```python
from build123d import *

# Parameters (mm, degrees)
F0_W     = 400
F0_H     = 1000
F0_W_2   = 250
F0_H_2   = 625
F0_H_3   = 150
F1_DEPTH = 50
F3_DEPTH = 400


with BuildPart() as f1:
    # F0 (on Front) → F1 (new body)
    with BuildSketch(Plane.XZ):
        with Locations((200, -500)):
            Rectangle(F0_W, F0_H)
        with Locations((200, -587.5)):
            Rectangle(F0_W_2, F0_H_2, mode=Mode.SUBTRACT)
        with Locations((200, -150)):
            Rectangle(F0_W_2, F0_H_3, mode=Mode.SUBTRACT)
    extrude(amount=-F1_DEPTH)

    # F2 (on face) → F3 (join)
    with BuildSketch(Plane.YZ.offset(400)):
        Polygon((-70, -1000), (0, -1000), (0, -962.657111), (-70, -975), align=None)
    extrude(amount=-F3_DEPTH)


solid = f1.part
```
Design review of the part built by this model. Coordinates are the model's own, in mm. A direction names the side the tool comes from. Give positions to 0.01 mm unless a question says otherwise; leave off trailing zeros. Order: outer loops, then holes, each group sorted by start corner. A loop starts at its lowest first (then second) coordinate and runs counter-clockwise, first axis right, second up. Notation, with made-up numbers: M 27.25,-20 L 75.25,-20 A37 ccw 75.25,16 Z; hole C 36,42.5 d2. An arc over 180 degrees is marked long. One line per question, with ' | ' between items. Start each with the question number.
Q1. The part is to be moulded in two halves that separate along X. For faces 4 (the face through (197, 25, 0)), 5 (the face through (0, 16, -493)), 6 (the face through (198, 25, -900)), say which applies: +X half, -X half, draft (parallel to the pull), parting line (faces both ways), or undercut.
Q2. For pin 1 Ø3 at (x, y) = (82.5, -58) entering from +Z; pin 2 Ø6 at (x, z) = (341, -542.5) entering from -Y; pin 3 Ø5 at (x, y) = (240, -28.5) entering from +Z, all flat-tipped, find the tip position at first contact; note any pin that passes through.
Q3. We need section A-A (z = -462.5). Write out the cut boundary in (x, y), plus the area to 3 significant figures.
Q4. Machinability: for faces 1 (the face through (400, 16, -493)), 2 (the face through (198, 25, -225)), 3 (the face through (331, 0, -475)), which of the approach directions +Z, -Z, +X, -X, +Y, -Y give a long, thin tool a straight path to every point of the face, cutting with its end or side? Answer none if there is none.
Q5. We need section D-D (x = 55). Write out the cut boundary in (y, z).
Q6. We need section B-B (y = 11.5). Write out the cut boundary in (x, z).
Q7. We need section C-C (x = 177). Write out the cut boundary in (y, z), plus the area to 3 significant figures.
Q8. For L1, parallel to Z at x = 285, y = 23.5; L2, parallel to X at y = 41.5, z = -795; L3, parallel to Y at x = 21, z = -94.5, list the stretches that pass through material, from the lowest coordinate up. Write a range as [from, to].
Returned:
1) face 4: draft | face 5: -X half | face 6: undercut
2) pin 1: z = -972.62 | pin 2: y = 0 | pin 3: z = -967.24
3) outline: M 0,0 L 75,0 L 75,50 L 0,50 Z; M 325,0 L 400,0 L 400,50 L 325,50 Z | area: 7,500 mm2
4) face 1: +Z, -Z, +X, +Y, -Y | face 2: +Y, -Y | face 3: +Z, +X, -X, -Y
5) outline: M -70,-1000 L 50,-1000 L 50,0 L 0,0 L 0,-962.66 L -70,-975 Z
6) outline: M 0,-1000 L 400,-1000 L 400,0 L 0,0 Z; hole M 75,-900 L 325,-900 L 325,-275 L 75,-275 Z; hole M 75,-225 L 325,-225 L 325,-75 L 75,-75 Z
7) outline: M -70,-1000 L 50,-1000 L 50,-900 L 0,-900 L 0,-962.66 L -70,-975 Z; M 0,-275 L 50,-275 L 50,-225 L 0,-225 Z; M 0,-75 L 50,-75 L 50,0 L 0,0 Z | area: 13,400 mm2
8) L1: [-1000, -900], [-275, -225], [-75, 0] | L2: [0, 75], [325, 400] | L3: [0, 50]
